```python
from build123d import *

# Parameters (mm, degrees)
SKETCH1_R           = 100
BOSS_EXTRUDE1_DEPTH = 25
SKETCH2_R           = 14
BOSS_EXTRUDE2_DEPTH = 80
SKETCH3_R           = 10
CUT_EXTRUDE1_DEPTH  = 4


with BuildPart() as part:
    # Sketch1 → Boss-Extrude1 (new body)
    with BuildSketch(Plane.XY):
        Circle(SKETCH1_R)
    extrude(amount=BOSS_EXTRUDE1_DEPTH)

    # Sketch2 → Boss-Extrude2 (add)
    with BuildSketch(Plane.XY.offset(25)):
        Circle(SKETCH2_R)
    extrude(amount=BOSS_EXTRUDE2_DEPTH)

    # Sketch3 → Cut-Extrude1 (cut)
    with BuildSketch(Plane(origin=(0, 0, 0), x_dir=(-1, 0, 0), z_dir=(0, 0, -1))):
        with Locations((0, 50)):
            Circle(SKETCH3_R)
    extrude(amount=-CUT_EXTRUDE1_DEPTH, mode=Mode.SUBTRACT)


solid = part.part
```
Check sheet for the modelled part. Datum: model origin and axes. Units: mm. A direction names the side the tool comes from. Coordinates: 2 decimals unless noted, no trailing zeros. Loops run counter-clockwise (first coordinate to the right, second up) from the corner with the lowest first, then second, coordinate; pieces in that order, holes last.
1) Gauge pin test, flat ends, axial feed: pin 1 (16 mm diameter, centred on x = 0, y = 50, fed in from -Z); pin 2 (1.5 mm diameter, centred on y = -47, z = 16, fed in from +X); pin 3 (4 mm diameter, centred on y = 43.5, z = 15.5, fed in from -X); pin 4 (10 mm diameter, centred on y = 66.5, z = 33.5, fed in from -X). Record the tip position at first contact, or that the pin passes through.
2) Release check for a two-part mould opening along X. For faces 1 (the face through (0, 0, 105)), 2 (the face through (95.38, 30.04, 12.32)), 3 (the face through (0, 50, 4)) record: released by +X, released by -X, zero draft, split by the parting line, or undercut.
3) Sectioned sample at B-B (y = 0). Record the boundary of the cut face in (x, z).
4) Sectioned sample at C-C (z = 21.5). Record the boundary of the cut face in (x, y).
5) Sectioned sample at D-D (y = 50). Record the boundary of the cut face in (x, z).
6) Sectioned sample at A-A (x = 0). Record the boundary of the cut face in (y, z), and give its area (3 significant figures).
7) Material ranges on probe 1 along Y at (x, z) = (0, 3); probe 2 along Z at (x, y) = (59, -18.5); probe 3 along Y at (x, z) = (-7, 5), recorded low to high.
8) Access from +Z, -Z, +X, -X, +Y, -Y to the whole of each face (thin tool, end or side, straight path). Record for faces 4 (the face through (-1, 1, 0)), 5 (the face through (2.17, 40.24, 1.97)), 6 (the face through (12.932, -5.362, 64.44)).
Check sheet entries:
1. pin 1: stops at z = 4
1. pin 2: stops at x = 88.66
1. pin 3: stops at x = -90.98
1. pin 4: passes through
2. face 1: zero draft
2. face 2: split by the parting line
2. face 3: undercut
3. outline: (-100, 0) - (100, 0) - (100, 25) - (14, 25) - (14, 105) - (-14, 105) - (-14, 25) - (-100, 25) - close
4. outline: circle Ø200 at (0, 0)
5. outline: (-86.6, 0) - (-10, 0) - (-10, 4) - (10, 4) - (10, 0) - (86.6, 0) - (86.6, 25) - (-86.6, 25) - close
6. outline: (-100, 0) - (40, 0) - (40, 4) - (60, 4) - (60, 0) - (100, 0) - (100, 25) - (14, 25) - (14, 105) - (-14, 105) - (-14, 25) - (-100, 25) - close
6. area: 7,160 mm2
7. probe 1: y = -100 to 40, 60 to 100
7. probe 2: z = 0 to 25
7. probe 3: y = -99.75 to 99.75
8. face 4: -Z, +X, -X, +Y, -Y
8. face 5: -Z
8. face 6: +Z
